Could you check a few things on this model? Use its own coordinates, in mm. Coordinates: 2 decimals unless noted, no trailing zeros. Loops run counter-clockwise (first coordinate to the right, second up) from the corner with the lowest first, then second, coordinate; pieces in that order, holes last. Notation, with made-up numbers: (-18, 3.25) -> (28, 3.25) arc R19 cw to (28, 26.25) -> close; hole circle Ø6 at (-28, 31). An arc over 180 degrees is marked (long way). One line per question, with ' | ' between items.
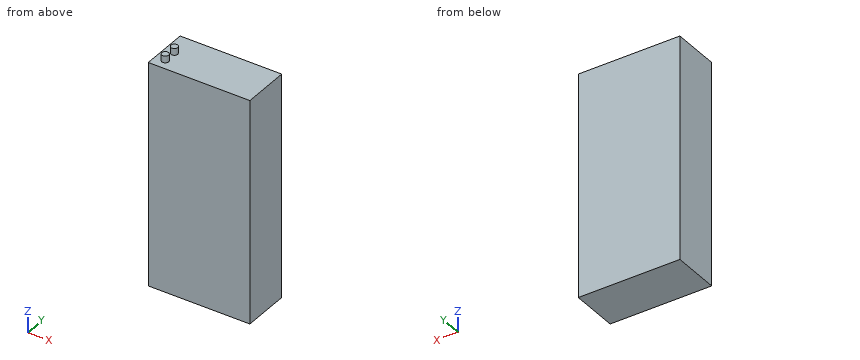
from build123d import *

# Parameters (mm, degrees)
SKETCH_1_W      = 150
SKETCH_1_H      = 70
EXTRUDE_1_DEPTH = 330
SKETCH_2_R      = 5
EXTRUDE_2_DEPTH = 10


with BuildPart() as part:
    # 草图1 → 凸台-拉伸1 (new body)
    with BuildSketch(Plane.XY):
        Rectangle(SKETCH_1_W, SKETCH_1_H)
    extrude(amount=EXTRUDE_1_DEPTH)

    # 草图2 → 凸台-拉伸2 (add)
    with BuildSketch(Plane.XY.offset(330)):
        with Locations((-60, 0)):
            Circle(SKETCH_2_R)
        with Locations((-60, -20)):
            Circle(SKETCH_2_R)
    extrude(amount=EXTRUDE_2_DEPTH)


solid = part.part
1) If we section it at C-C on x = 59: Please give me the cut outline in (y, z), and give its area (3 significant figures).
Data:
outline: (-35, 0) -> (35, 0) -> (35, 330) -> (-35, 330) -> close | area: 23,100 mm²
2) If we section it at B-B on y = -20: Please give me the cut outline in (x, z), and give its area (3 significant figures).
Data:
outline: (-75, 0) -> (75, 0) -> (75, 330) -> (-55, 330) -> (-55, 340) -> (-65, 340) -> (-65, 330) -> (-75, 330) -> close | area: 49,600 mm²
3) If we section it at A-A on x = -60: Please give me the cut outline in (y, z).
Data:
outline: (-35, 0) -> (35, 0) -> (35, 330) -> (5, 330) -> (5, 340) -> (-5, 340) -> (-5, 330) -> (-15, 330) -> (-15, 340) -> (-25, 340) -> (-25, 330) -> (-35, 330) -> close
4) I need wall thicknesses on line 1 along Z through (x, y) = (35, 17). Which ranges of the line are inside material? Lowest first, please. Write a range as from..to.
Data:
line 1: 0..330
